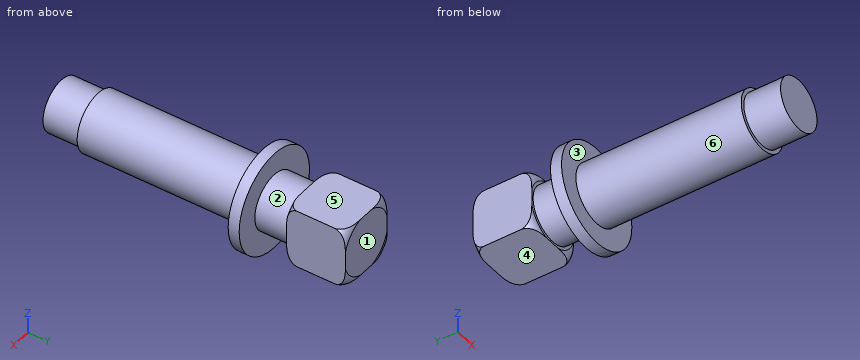
from build123d import *

# Parameters (mm, degrees)
SKETCH2_W           = 16
SKETCH2_H           = 16
BOSS_EXTRUDE1_DEPTH = 16


with BuildPart() as part:
    # Sketch1 → Revolve1 (revolve)
    with BuildSketch(Plane.XY):
        Polygon((0, 0), (7, 0), (7, 10), (8, 10), (8, 55), (13.5, 55), (13.5, 58), (7.5, 58), (7.5, 67), (0, 67), align=None)
    revolve(axis=Axis((0, 0, 0), (0, 1, 0)))

    # Sketch2 → Boss-Extrude1 (add)
    with BuildSketch(Plane(origin=(0, 67, 0), x_dir=(1, 0, 0), z_dir=(0, 1, 0))):
        Rectangle(SKETCH2_W, SKETCH2_H)
    extrude(amount=BOSS_EXTRUDE1_DEPTH)

    # Sketch4 → Cut-Revolve1 (revolve, cut)
    with BuildSketch(Plane(origin=(0, 0, 0), x_dir=(0.707106781, 0, -0.707106781), z_dir=(0.707106781, 0, 0.707106781))):
        with BuildLine():
            Line((11.313708499, 83), (8.313708499, 83))
            ThreePointArc((8.313708499, 83), (10.435028843, 82.121320344), (11.313708499, 80))
            Line((11.313708499, 80), (11.313708499, 83))
        make_face()
        with BuildLine():
            Line((11.313708499, 67), (8.313708499, 67))
            ThreePointArc((8.313708499, 67), (10.435028843, 67.878679656), (11.313708499, 70))
            Line((11.313708499, 70), (11.313708499, 67))
        make_face()
    revolve(axis=Axis((0, 66.528771151, 0), (0, 1, 0)), mode=Mode.SUBTRACT)


solid = part.part
Can you work these out from the model? Positions are in its coordinate system, mm. Face numbers are marked on the shaded views. A direction names the side the tool comes from. Coordinates: 2 decimals unless noted, no trailing zeros. Loops run counter-clockwise (first coordinate to the right, second up) from the corner with the lowest first, then second, coordinate; pieces in that order, holes last. Notation, with made-up numbers: (13.5, 11) - (17.5, 11) arc R33 ccw to (17.5, 47) - close; hole circle Ø10 at (-18, -20.75). An arc over 180 degrees is marked (long way). Answer as a JSON object with one key per item and string values. Group by question number.
Item 1: If we section it at A-A (z = 0): List the corners of the cut face in (x, y) for me, plus the area to 3 significant figures.
Item 2: If we mould it in two halves opening along Y, with no side actions, what happens to the marked faces 1, 2 and 3? For each: released by +Y, released by -Y, zero draft, split by the parting line, or undercut.
Item 3: If we section it at C-C (y = 66): List the corners of the cut face in (x, z) for me.
Item 4: For pin 1 (1 mm diameter, centred on y = 33.5, z = -4.5, fed in from -X); pin 2 (8 mm diameter, centred on y = 60, z = 6.5, fed in from -X); pin 3 (5 mm diameter, centred on x = -2, z = 4, fed in from -Y); pin 4 (13 mm diameter, centred on y = 79, z = -2.5, fed in from +X), each with a flat end and sliding along its axis, tell me the tip position at first contact or that it passes through.
Item 5: If I drill on L1, parallel to X at y = 79, z = -3.5; L2, parallel to Y at x = 0.75, z = -7, over which ranges is the centre line in solid material (lowest first)? Write a range as from..to.
Item 6: If we section it at D-D (y = 34): List the corners of the cut face in (x, z) for me, plus the area to 3 significant figures.
Item 7: On a 3-axis mill with a long thin cutter (end or side, diameter ignored), from which of +Z, -Z, +X, -X, +Y, -Y can I reach the whole of each face in a straight line? I mean the marked faces 4, 5 and 6. Say none if no direction works.
Item 8: If we section it at B-B (x = 0): List the corners of the cut face in (y, z) for me.
Returned:
{
 "1": {"outline": "(-13.5, 55) - (-8, 55) - (-8, 10) - (-7, 10) - (-7, 0) - (7, 0) - (7, 10) - (8, 10) - (8, 55) - (13.5, 55) - (13.5, 58) - (7.5, 58) - (7.5, 67) - (8, 67) - (8, 83) - (-8, 83) - (-8, 67) - (-7.5, 67) - (-7.5, 58) - (-13.5, 58) - close", "area": "1,330 mm²"},
 "2": {"face 1": "released by +Y", "face 2": "undercut", "face 3": "released by -Y"},
 "3": {"outline": "circle Ø15 at (0, 0)"},
 "4": {"pin 1": "stops at x = -6.93", "pin 2": "stops at x = -13.15", "pin 3": "stops at y = 0", "pin 4": "stops at x = 8"},
 "5": {"L1": "x = -8..8", "L2": "y = 10..83"},
 "6": {"outline": "circle Ø16 at (0, 0)", "area": "201 mm²"},
 "7": {"face 4": "-Z, +X, -X, +Y", "face 5": "+Z, +X, -X, +Y", "face 6": "-Y"},
 "8": {"outline": "(0, -7) - (10, -7) - (10, -8) - (55, -8) - (55, -13.5) - (58, -13.5) - (58, -7.5) - (67, -7.5) - (67, -8) - (83, -8) - (83, 8) - (67, 8) - (67, 7.5) - (58, 7.5) - (58, 13.5) - (55, 13.5) - (55, 8) - (10, 8) - (10, 7) - (0, 7) - close"}
}
